from build123d import *

# Parameters (mm, degrees)
F1_DEPTH = 152.4
F2_R     = 25.4
F3_R     = 25.4
F4_R     = 25.4
F5_R     = 25.4


# Not quite as in the source:
# - a feature names something its author has since deleted; it is built from what else it names


with BuildPart() as f1:
    # F0 (on Right) → F1 (new body)
    with BuildSketch(Plane.YZ):
        with BuildLine():
            Line((0, -63.5), (0, 0))
            Line((0, 0), (-50.2625516508, 42.1752885522))
            ThreePointArc((-50.2625516508, 42.1752885522), (-126.6574881065, 86.2819256796), (-213.5306045112, 101.6))
            Line((-213.5306045112, 101.6), (-254, 101.6))
            Line((-254, 101.6), (-254, 38.1))
            Line((-254, 38.1), (-224.2420489686, 38.1))
            ThreePointArc((-224.2420489686, 38.1), (-204.8017306044, 34.2330802516), (-188.3210244843, 23.2210244843))
            Line((-188.3210244843, 23.2210244843), (-179.9789755157, 14.8789755157))
            ThreePointArc((-179.9789755157, 14.8789755157), (-168.9669197484, -1.6017306044), (-165.1, -21.0420489686))
            Line((-165.1, -21.0420489686), (-165.1, -63.5))
            Line((-165.1, -63.5), (0, -63.5))
        make_face()
    extrude(amount=F1_DEPTH)

    # F2
    f2_edges = [f1.edges().sort_by_distance(p)[0] for p in [
        (0, -233.765302, 101.6),
        (0, 0, -31.75),
    ]]
    fillet(f2_edges, radius=F2_R)

    # F3
    f3_edges = [f1.edges().sort_by_distance(p)[0] for p in [
        (0, -165.1, -42.271024),
    ]]
    fillet(f3_edges, radius=F3_R)

    # F4
    f4_edges = [f1.edges().sort_by_distance(p)[0] for p in [
        (152.4, -165.1, -42.271024),
    ]]
    fillet(f4_edges, radius=F4_R)

    # F5
    f5_edges = [f1.edges().sort_by_distance(p)[0] for p in [
        (152.4, -233.765302, 101.6),
        (152.4, 0, -31.75),
    ]]
    fillet(f5_edges, radius=F5_R)

    # F9: sweep along a path in F8
    with BuildLine(Plane.YZ.offset(76.2)) as f9_path:
        Line((-254, 69.85), (-213.5306045112, 69.85))
        ThreePointArc((-213.5306045112, 69.85), (-137.5166276571, 56.4466849697), (-70.6710582584, 17.8533774832))
        Line((-70.6710582584, 17.8533774832), (74.6758873088, -104.1071909349))
    # F6 (on face) → F9 (sweep, cut)
    with BuildSketch(Plane.XZ.offset(254)):
        with BuildLine():
            Line((25.4, 41.91), (127, 41.91))
            ThreePointArc((127, 41.91), (142.2664354058, 48.2335645942), (148.59, 63.5))
            Line((148.59, 63.5), (148.59, 76.2))
            ThreePointArc((148.59, 76.2), (142.2664354058, 91.4664354058), (127, 97.79))
            Line((127, 97.79), (25.4, 97.79))
            ThreePointArc((25.4, 97.79), (10.1335645942, 91.4664354058), (3.81, 76.2))
            Line((3.81, 76.2), (3.81, 63.5))
            ThreePointArc((3.81, 63.5), (10.1335645942, 48.2335645942), (25.4, 41.91))
        make_face()
    sweep(path=f9_path.line, mode=Mode.SUBTRACT)


solid = f1.part
Model file for the job. Use its own axes, mm. A direction names the side the tool comes from. Round coordinates to 2 decimals unless told otherwise and drop trailing zeros. Loops run counter-clockwise (first coordinate to the right, second up) from the corner with the lowest first, then second, coordinate; pieces in that order, holes last. Notation, with made-up numbers: (60, -10) -> (73, -10) arc R16 ccw to (73, -3) -> close; hole circle Ø6 at (-20.5, -35). An arc over 180 degrees is marked (long way). Answer as CSV lines item,"result". Start each with the question number.
1) Slice it at A-A (x = 89). List the corners of the cut face in (y, z).
2) Mould opens along Y. For faces 1 (the face through (142.098, -29.002, 11.325)), 2 (the face through (75, -165.1, -42)), 3 (the face through (0, -116, 7)) say: +Y half, -Y half, draft (parallel to the pull), parting line (faces both ways), or undercut.
3) Probe line 1 along X through (y, z) = (-232, 67); line 2 along Z through (x, y) = (94.5, -230); line 3 along Z through (x, y) = (120, -37.5). List the from-to ranges inside material, lowest first.
4) Pin check, flat tips, straight feed: P1, Ø8, axis at x = 116.5, y = -158.5, coming from the +Z side; P2, Ø5, axis at x = 77.5, y = -185, coming from the -Z side; P3, Ø12.5, axis at x = 54, z = -41.5, coming from the -Y side. Stop position of each tip, or through.
5) Tool access for faces 4 (the face through (75, -239, 38.1)), 5 (the face through (142.43, -233.48, 48.4)), 6 (the face through (145.16, -234.05, 93.96)), 7 (the face through (7.24, -238.91, 45.74)), 8 (the face through (76.911, -25.987, 16.832)): list every direction of +Z, -Z, +X, -X, +Y, -Y with a clear straight run to the whole face (end or side of a thin tool).
Filled in:
1,outline,"(-254, 38.1) -> (-224.24, 38.1) arc R50.8 cw to (-188.32, 23.22) -> (-179.98, 14.88) arc R50.8 cw to (-165.1, -21.04) -> (-165.1, -63.5) -> (-17.18, -63.5) -> (-88.63, -3.55) arc R194.31 ccw to (-213.53, 41.91) -> (-254, 41.91) -> close; (-254, 97.79) -> (-213.53, 97.79) arc R250.19 cw to (-52.71, 39.26) -> (0, -4.97) -> (0, 0) -> (-50.26, 42.18) arc R254 ccw to (-213.53, 101.6) -> (-254, 101.6) -> close"
2,face 1,"undercut"
2,face 2,"-Y half"
2,face 3,"draft"
3,line 1,"x = 0 to 3.81, 148.59 to 152.4"
3,line 2,"z = 38.1 to 41.91, 97.79 to 101.6"
3,line 3,"z = -63.5 to -46.45, 26.49 to 31.47"
4,P1,"stops at z = 96.42"
4,P2,"stops at z = 17.4"
4,P3,"stops at y = -165.1"
5,face 4,"-Z, +X, -X, -Y"
5,face 5,"-Y"
5,face 6,"+Z, +X, +Y, -Y"
5,face 7,"-Z, -X, -Y"
5,face 8,"none"
